from build123d import *

# Parameters (mm, degrees)
EXTRUDE_THIN1_START = -2.5
EXTRUDE_THIN1_DEPTH = 5


with BuildPart() as part:
    # Sketch2 → Extrude-Thin1 (new, symmetric)
    with BuildSketch(Plane.XY.offset(EXTRUDE_THIN1_START)):
        with BuildLine():
            Line((-285.070155578, -13.000246093), (0.077171136, -10.999729297))
            ThreePointArc((0.077171136, -10.999729297), (10.999932323, 0.038585806), (0, 11))
            Line((0, 11), (-316, 11))
            ThreePointArc((-316, 11), (-323.762020666, 7.794295041), (-326.999905306, 0.045642761))
            Line((-326.999905306, 0.045642761), (-327.149905306, -36.104357239))
            ThreePointArc((-327.149905306, -36.104357239), (-318.900034366, -46.800695329), (-306.503020259, -41.435431097))
            Line((-306.503020259, -41.435431097), (-293.769981583, -18.195062639))
            ThreePointArc((-293.769981583, -18.195062639), (-290.126747116, -14.414170744), (-285.070155578, -13.000246093))
        make_face()
        with BuildLine():
            Line((-285.073663357, -12.500258398), (0.073663357, -10.499741602))
            ThreePointArc((0.073663357, -10.499741602), (10.499935399, 0.036831905), (0, 10.5))
            Line((0, 10.5), (-316, 10.5))
            ThreePointArc((-316, 10.5), (-323.409201545, 7.440008903), (-326.49990961, 0.04356809))
            Line((-326.49990961, 0.04356809), (-326.64990961, -36.10643191))
            ThreePointArc((-326.64990961, -36.10643191), (-318.775032804, -46.316572814), (-306.941519338, -41.195184229))
            Line((-306.941519338, -41.195184229), (-294.208480662, -17.954815771))
            ThreePointArc((-294.208480662, -17.954815771), (-290.383084472, -13.984879282), (-285.073663357, -12.500258398))
        make_face(mode=Mode.SUBTRACT)
    extrude(amount=EXTRUDE_THIN1_DEPTH, both=True)


solid = part.part
Could you check a few things on this model? Use its own coordinates, in mm. A direction names the side the tool comes from. Give positions to 0.01 mm unless a question says otherwise; leave off trailing zeros. Order: outer loops, then holes, each group sorted by start corner. A loop starts at its lowest first (then second) coordinate and runs counter-clockwise, first axis right, second up. Notation, with made-up numbers: (46, 28.5) - (73, 28.5) arc R27 cw to (73, 47.5) - close; hole circle Ø9 at (14, 5). An arc over 180 degrees is marked (long way). One line per item, written item: value. Start each with the question number.
1. Imagine slicing it at B-B on x = -115.5. List the corners of the cut face in (y, z) for me.
2. If I drill on probe 1 along Y at (x, z) = (-262.5, 2.25); probe 2 along Y at (x, z) = (-302.5, 1.75); probe 3 along X at (y, z) = (-35, -3), over which ranges is the centre line in solid material (lowest first)?
3. Thinking about a two-plate mould opening in X: for faces 3 (the face through (11, 0, -2)), 4 (the face through (-319.097, -46.748, -2.43)), 5 (the face through (-300.664, -29.738, -2.43)), which applies, +X half, -X half, draft (parallel to the pull), parting line (faces both ways), or undercut?
4. Imagine slicing it at A-A on z = 0.5. List the corners of the cut face in (x, y) for me, plus the area to 3 significant figures.
5. For faces 1 (the face through (-323.676, 7.879, -2.43)), 2 (the face through (-156, 10.5, -2)), which set-ups out of +Z, -Z, +X, -X, +Y, -Y let a thin tool reach every point of the face, with its end or its side?
6. For P1, Ø3, axis at x = -224.5, z = -5, coming from the -Y side; P2, Ø5, axis at y = -37, z = -2, coming from the +X side; P3, Ø1.5, axis at y = -30, z = -5, coming from the -X side, each with a flat end and sliding along its axis, tell me the tip position at first contact or that it passes through.
7. Imagine slicing it at C-C on y = 6. List the corners of the cut face in (x, z) for me.
Values:
1. outline: (-11.81, -7.5) - (-11.31, -7.5) - (-11.31, 2.5) - (-11.81, 2.5) - close; (10.5, -7.5) - (11, -7.5) - (11, 2.5) - (10.5, 2.5) - close
2. probe 1: -12.84 to -12.34, 10.5 to 11
2. probe 2: -34.13 to -33.09, 10.5 to 11
2. probe 3: -327.15 to -326.65, -303.55 to -302.98
3. face 3: +X half
3. face 4: parting line
3. face 5: undercut
4. outline: (-327.15, -36.1) arc R11 ccw to (-306.5, -41.44) - (-293.77, -18.2) arc R10 cw to (-285.07, -13) - (0.08, -11) arc R11 ccw to (0, 11) - (-316, 11) arc R11 ccw to (-327, 0.05) - close; hole (-326.65, -36.11) arc R10.5 ccw to (-306.94, -41.2) - (-294.21, -17.95) arc R10.5 cw to (-285.07, -12.5) - (0.07, -10.5) arc R10.5 ccw to (0, 10.5) - (-316, 10.5) arc R10.5 ccw to (-326.5, 0.04) - close
4. area: 377 mm²
5. face 1: +Z, -Z, -X, +Y
5. face 2: +Z, -Z
6. P1: y = -12.59
6. P2: x = -302.7
6. P3: x = -327.13
7. outline: (-325.22, -7.5) - (-324.62, -7.5) - (-324.62, 2.5) - (-325.22, 2.5) - close; (8.62, -7.5) - (9.22, -7.5) - (9.22, 2.5) - (8.62, 2.5) - close
